Answer from the drawing. Dimensions are ordinates in mm from the lowest x, y and z of the part. Give positions to 0.01 mm unless a question says otherwise; leave off trailing zeros. Order: outer loops, then holes, each group sorted by start corner. A loop starts at its lowest first (then second) coordinate and runs counter-clockwise, first axis right, second up.
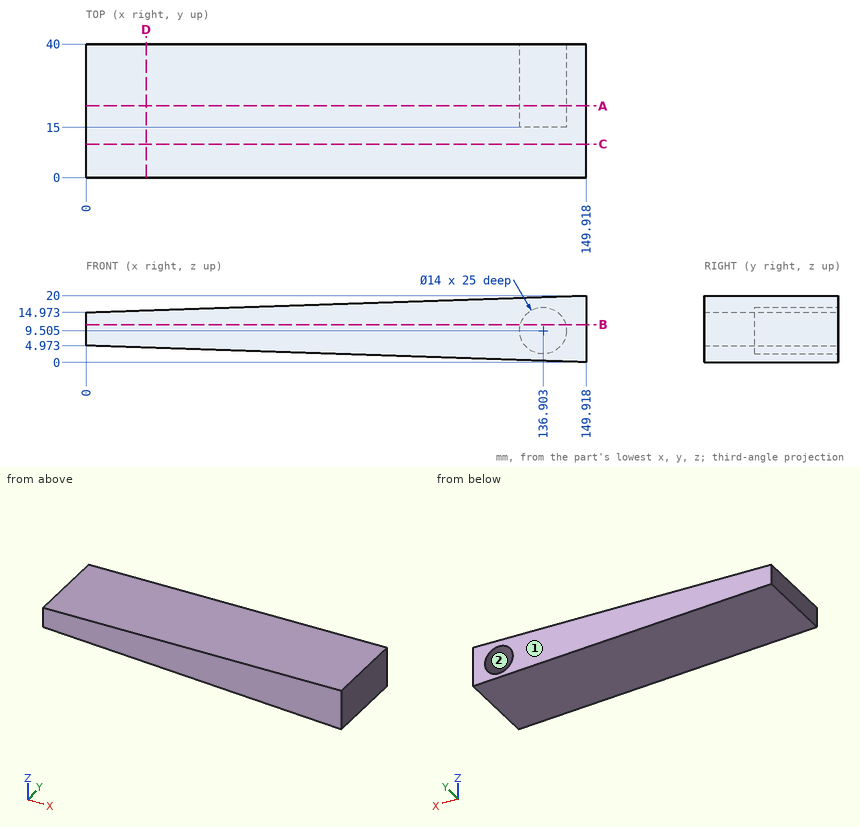
1) The part is cut by section C-C on y = 10. Determine the outline of the cut face in (x, z), and give its area (3 significant figures).
Final values:
outline: (0, 4.97) - (149.92, 0) - (149.92, 20) - (0, 14.97) - close
area: 2,250 mm2
2) The part is cut by section A-A on y = 21.5. Determine the outline of the cut face in (x, z) (1 decimal).
Final values:
outline: (0, 5) - (149.9, 0) - (149.9, 20) - (0, 15) - close; hole circle Ø14 at (136.9, 9.5)
3) The part is cut by section D-D on x = 18. Determine the outline of the cut face in (y, z), and give its area (3 significant figures).
Final values:
outline: (0, 4.38) - (40, 4.38) - (40, 15.58) - (0, 15.58) - close
area: 448 mm2
4) Given pin 1 (7 mm diameter, centred on x = 139.5, z = 8.5, fed in from +Y); pin 2 (2 mm diameter, centred on x = 23.5, y = 14, fed in from -Z); pin 3 (1 mm diameter, centred on x = 76, y = 22, fed in from -Z) (1 decimal), each flat-ended and moving along its own axis, determine where each tip first touches the part or whether it passes through.
Final values:
pin 1: stops at y = 15
pin 2: stops at z = 4.16
pin 3: stops at z = 2.4
5) For a pull along Z with two mould halves and no side action, classify the marked faces 1 and 2 as released by +Z, released by -Z, zero draft, split by the parting line, or undercut.
Final values:
face 1: zero draft
face 2: undercut
6) The part is cut by section B-B on z = 11.25. Determine the outline of the cut face in (x, y) (1 decimal).
Final values:
outline: (0, 0) - (149.9, 0) - (149.9, 40) - (143.7, 40) - (143.7, 15) - (130.1, 15) - (130.1, 40) - (0, 40) - close
7) Consider L1, parallel to X at y = 20.5, z = 8.25; L2, parallel to X at y = 19, z = 8.75 (1 decimal); L3, parallel to Z at x = 17, y = 20.5. Determine where each line is inside the solid, lowest interval first.
Final values:
L1: x = 0 to 130.02, 143.79 to 149.92
L2: x = 0 to 129.9, 143.9 to 149.9
L3: z = 4.41 to 15.54
